```python
from build123d import *

# Parameters (mm, degrees)
SKETCH1_W           = 127.381
SKETCH1_H           = 77.0636
SKETCH1_R           = 1.651
SKETCH1_R_2         = 0.79375
SKETCH1_R_3         = 1.7145
SKETCH1_R_4         = 1.659299133
BOSS_EXTRUDE1_DEPTH = 1.5875
FILLET1_R           = 3.175


with BuildPart() as part:
    # Sketch1 → Boss-Extrude1 (new body)
    with BuildSketch(Plane.XY):
        with Locations((54.1655, 38.5318)):
            Rectangle(SKETCH1_W, SKETCH1_H)
        with Locations((-6.35, 6.35)):
            Circle(SKETCH1_R, mode=Mode.SUBTRACT)
        with Locations((10.3251, 2.6924)):
            Circle(SKETCH1_R_2, mode=Mode.SUBTRACT)
        with Locations((24.2443, 2.6924)):
            Circle(SKETCH1_R_2, mode=Mode.SUBTRACT)
        with Locations((18.3261, 10.9093)):
            Circle(SKETCH1_R_3, mode=Mode.SUBTRACT)
        with Locations((32.2453, 2.6924)):
            Circle(SKETCH1_R_2, mode=Mode.SUBTRACT)
        with Locations((54.1655, 2.6924)):
            Circle(SKETCH1_R_2, mode=Mode.SUBTRACT)
        with Locations((40.2463, 10.9093)):
            Circle(SKETCH1_R_3, mode=Mode.SUBTRACT)
        with Locations((-6.35, 27.1018)):
            Circle(SKETCH1_R_4, mode=Mode.SUBTRACT)
        with Locations((-6.35, 30.9118)):
            Circle(SKETCH1_R_4, mode=Mode.SUBTRACT)
        with Locations((-6.35, 34.7218)):
            Circle(SKETCH1_R_4, mode=Mode.SUBTRACT)
        with Locations((66.1543, 2.6924)):
            Circle(SKETCH1_R_2, mode=Mode.SUBTRACT)
        with Locations((76.0857, 2.6924)):
            Circle(SKETCH1_R_2, mode=Mode.SUBTRACT)
        with Locations((62.1665, 10.9093)):
            Circle(SKETCH1_R_3, mode=Mode.SUBTRACT)
        with Locations((84.0867, 10.9093)):
            Circle(SKETCH1_R_3, mode=Mode.SUBTRACT)
        with Locations((98.0059, 2.6924)):
            Circle(SKETCH1_R_2, mode=Mode.SUBTRACT)
        with Locations((114.681, 6.35)):
            Circle(SKETCH1_R, mode=Mode.SUBTRACT)
        with Locations((106.0069, 10.9093)):
            Circle(SKETCH1_R_3, mode=Mode.SUBTRACT)
        with Locations((-6.35, 38.5318)):
            Circle(SKETCH1_R_4, mode=Mode.SUBTRACT)
        with Locations((-6.35, 42.3418)):
            Circle(SKETCH1_R_4, mode=Mode.SUBTRACT)
        with Locations((-6.35, 46.1518)):
            Circle(SKETCH1_R_4, mode=Mode.SUBTRACT)
        with Locations((-6.35, 49.9618)):
            Circle(SKETCH1_R_4, mode=Mode.SUBTRACT)
        with Locations((2.3241, 66.1543)):
            Circle(SKETCH1_R_3, mode=Mode.SUBTRACT)
        with Locations((24.2443, 66.1543)):
            Circle(SKETCH1_R_3, mode=Mode.SUBTRACT)
        with Locations((-6.35, 70.7136)):
            Circle(SKETCH1_R, mode=Mode.SUBTRACT)
        with Locations((10.3251, 74.3712)):
            Circle(SKETCH1_R_2, mode=Mode.SUBTRACT)
        with Locations((18.3261, 74.4347)):
            Circle(SKETCH1_R_2, mode=Mode.SUBTRACT)
        with Locations((46.1645, 66.1543)):
            Circle(SKETCH1_R_3, mode=Mode.SUBTRACT)
        with Locations((32.2453, 74.3712)):
            Circle(SKETCH1_R_2, mode=Mode.SUBTRACT)
        with Locations((54.1655, 74.3712)):
            Circle(SKETCH1_R_2, mode=Mode.SUBTRACT)
        with Locations((68.0847, 66.1543)):
            Circle(SKETCH1_R_3, mode=Mode.SUBTRACT)
        with Locations((90.0049, 66.1543)):
            Circle(SKETCH1_R_3, mode=Mode.SUBTRACT)
        with Locations((60.2361, 74.4347)):
            Circle(SKETCH1_R_2, mode=Mode.SUBTRACT)
        with Locations((76.0857, 74.3712)):
            Circle(SKETCH1_R_2, mode=Mode.SUBTRACT)
        with Locations((98.0059, 74.3712)):
            Circle(SKETCH1_R_2, mode=Mode.SUBTRACT)
        with Locations((102.1461, 74.4347)):
            Circle(SKETCH1_R_2, mode=Mode.SUBTRACT)
        with Locations((106.0069, 74.4347)):
            Circle(SKETCH1_R_2, mode=Mode.SUBTRACT)
        with Locations((114.681, 70.7136)):
            Circle(SKETCH1_R, mode=Mode.SUBTRACT)
    extrude(amount=BOSS_EXTRUDE1_DEPTH)

    # Fillet1
    fillet1_edges = [part.edges().sort_by_distance(p)[0] for p in [
        (-9.525, 77.0636, 0.79375),
        (117.856, 77.0636, 0.79375),
        (117.856, 0, 0.79375),
        (-9.525, 0, 0.79375),
    ]]
    fillet(fillet1_edges, radius=FILLET1_R)


solid = part.part
```
The listing builds one solid part. Answer for the finished solid, in the listing's coordinates (mm). Round coordinates to 2 decimals unless told otherwise and drop trailing zeros. Loops run counter-clockwise (first coordinate to the right, second up) from the corner with the lowest first, then second, coordinate; pieces in that order, holes last.
Q1. Section B-B, the plane z = 0.3 is taken. Count the separate pieces of the cut face and the enclosed holes in it, then the cut area to 3 significant figures.
Q2. Section A-A, the plane y = 6.35 is taken. Determine the outline of the cut face in (x, z) (1 decimal).
Q3. Find the intervals of material crossed by line 1 (X direction, y = 70.5, z = 0.4) (3 decimals); line 2 (X direction, y = 5, z = 0.3) (3 decimals); line 3 (X direction, y = 50, z = 0.15) (3 decimals), in increasing order.
Q4. Given pin 1 Ø4 at (x, y) = (-6.35, 46.15) entering from -Z, flat-ended and moving along its own axis, determine where the tip first touches the part or whether it passes through.
Q5. For a pull along X with two mould halves and no side action, classify faces 1 (the face through (-6.566, 43.987, 0.783)), 2 (the face through (53, 39, 1.588)), 3 (the face through (-8.62, 0.955, 0.805)) as released by +X, released by -X, zero draft, split by the parting line, or undercut.
Completed:
1. separate pieces: 1
1. enclosed holes: 37
1. area: 9,590 mm2
2. outline: (-9.5, 0) - (-8, 0) - (-8, 1.6) - (-9.5, 1.6) - close; (-4.7, 0) - (113, 0) - (113, 1.6) - (-4.7, 1.6) - close; (116.3, 0) - (117.9, 0) - (117.9, 1.6) - (116.3, 1.6) - close
3. line 1: x = -9.525 to -7.987, -4.713 to 113.044, 116.318 to 117.856
3. line 2: x = -9.525 to -7.3, -5.4 to 113.731, 115.631 to 117.856
3. line 3: x = -9.525 to -8.009, -4.691 to 117.856
4. pin 1: stops at z = 0
5. face 1: undercut
5. face 2: zero draft
5. face 3: released by -X
